Source: CAD feature listing. Evaluate the final solid. Frame: model axes, mm. A direction names the side the tool comes from. Give positions to 0.01 mm unless a question says otherwise; leave off trailing zeros. Write each loop counter-clockwise with the first axis right and the second up, starting at its lowest first coordinate (ties: lowest second). Pieces come first, ordered by that corner, then holes. Notation, with made-up numbers: (40, 20.25) -> (67, 20.25) arc R31 cw to (67, 51.25) -> close; hole circle Ø5 at (3, 29.5). An arc over 180 degrees is marked (long way). Write item = value, one per line.
from build123d import *

# Parameters (mm, degrees)
SKETCH_R        = 1.95
SKETCH_W        = 6.8
SKETCH_H        = 46.08113
PAD_DEPTH       = 3
SKETCH001_W     = 22
SKETCH001_H     = 72
PAD001_DEPTH    = 6.5
SKETCH002_W     = 8
SKETCH002_H     = 40
PAD002_DEPTH    = 7.5
SKETCH003_R     = 6.1
POCKET_DEPTH    = 3.5
SKETCH004_R     = 3
POCKET001_DEPTH = 6.5
CHAMFER_SIZE    = 3
CHAMFER001_SIZE = 0.5


with BuildPart() as part:
    # Sketch → Pad (new body)
    with BuildSketch(Plane.XY):
        Polygon((54.045437, 24.98), (101.633751, 24.98), (101.633751, -24.98), (54.045437, -24.98), (43.025437, -36), (0, -36), (0, 36), (43.025437, 36), align=None)
        with Locations((42.6, 21.78)):
            Circle(SKETCH_R, mode=Mode.SUBTRACT)
        with Locations((42.6, -21.78)):
            Circle(SKETCH_R, mode=Mode.SUBTRACT)
        with Locations((96.7, 21.78)):
            Circle(SKETCH_R, mode=Mode.SUBTRACT)
        with Locations((96.7, -21.78)):
            Circle(SKETCH_R, mode=Mode.SUBTRACT)
        with Locations((35.4, 0)):
            Rectangle(SKETCH_W, SKETCH_H, mode=Mode.SUBTRACT)
    extrude(amount=PAD_DEPTH)

    # Sketch001 → Pad001 (join)
    with BuildSketch(Plane.XY):
        with Locations((11, 0)):
            Rectangle(SKETCH001_W, SKETCH001_H)
    extrude(amount=PAD001_DEPTH)

    # Sketch002 → Pad002 (join)
    with BuildSketch(Plane.XY):
        with Locations((14, 0)):
            Rectangle(SKETCH002_W, SKETCH002_H)
    extrude(amount=PAD002_DEPTH)

    # Sketch003 → Pocket (cut)
    with BuildSketch(Plane.XY):
        with Locations((14, 25)):
            Circle(SKETCH003_R)
        with Locations((14, -25)):
            Circle(SKETCH003_R)
    extrude(amount=POCKET_DEPTH, mode=Mode.SUBTRACT)

    # Sketch004 → Pocket001 (cut)
    with BuildSketch(Plane.XY):
        with Locations((14, 25)):
            Circle(SKETCH004_R)
        with Locations((14, -25)):
            Circle(SKETCH004_R)
    extrude(amount=POCKET001_DEPTH, mode=Mode.SUBTRACT)

    # Chamfer
    chamfer_edges = [part.edges().sort_by_distance(p)[0] for p in [
        (101.633751, -24.98, 1.5),
        (101.633751, 24.98, 1.5),
        (22, 36, 4.75),
        (0, 36, 1.5),
        (0, 36, 4.75),
        (0, -36, 4.75),
        (0, -36, 1.5),
        (22, -36, 4.75),
    ]]
    chamfer(chamfer_edges, length=CHAMFER_SIZE)

    # Chamfer001
    chamfer001_edges = [part.edges().sort_by_distance(p)[0] for p in [
        (48.535437, 30.49, 3),
        (76.339594, 24.98, 3),
        (100.133751, 23.48, 3),
        (101.633751, 0, 3),
        (100.133751, -23.48, 3),
        (76.339594, -24.98, 3),
        (76.339594, -24.98, 0),
        (48.535437, -30.49, 3),
        (48.535437, -30.49, 0),
        (32.512719, -36, 0),
        (32.512719, -36, 3),
        (1.5, -34.5, 0),
        (0, 0, 0),
        (1.5, 34.5, 6.5),
        (32.512719, 36, 3),
        (11, 36, 6.5),
        (1.5, 34.5, 0),
        (12.5, 36, 0),
        (100.133751, -23.48, 0),
        (76.339594, 24.98, 0),
        (22, 0, 6.5),
        (44.55, 21.78, 1.5),
        (20.5, 34.5, 6.5),
        (20.5, -36, 3),
        (0, 0, 6.5),
        (12.5, -36, 0),
        (20.5, 36, 3),
        (32.512719, 36, 0),
        (48.535437, 30.49, 0),
        (100.133751, 23.48, 0),
        (101.633751, 0, 0),
        (20.5, -34.5, 6.5),
        (11, -36, 6.5),
        (1.5, -34.5, 6.5),
    ]]
    chamfer(chamfer001_edges, length=CHAMFER001_SIZE)


solid = part.part
(1) Section query A-A (z = 5). Return loops of the section in (x, y).
Values follow:
outline = (0, -33) -> (3, -36) -> (19, -36) -> (22, -33) -> (22, 33) -> (19, 36) -> (3, 36) -> (0, 33) -> close; hole circle Ø6 at (14, -25); hole circle Ø6 at (14, 25)
(2) Section query C-C (y = -27). Return loops of the section in (x, z), plus the area to 3 significant figures.
Values follow:
outline = (0, 0.5) -> (0.5, 0) -> (8.24, 0) -> (8.24, 3.5) -> (11.76, 3.5) -> (11.76, 6.5) -> (0.5, 6.5) -> (0, 6) -> close; (16.24, 3.5) -> (19.76, 3.5) -> (19.76, 0) -> (51.32, 0) -> (52.03, 0.5) -> (52.03, 2.5) -> (51.32, 3) -> (22, 3) -> (22, 6) -> (21.5, 6.5) -> (16.24, 6.5) -> close
area = 179 mm2
(3) First-contact query: pin 1 (12 mm diameter, centred on x = 43.5, y = -4.5, fed in from +Z); pin 2 (7.5 mm diameter, centred on x = 14, y = 25, fed in from +Z); pin 3 (3 mm diameter, centred on y = -2.5, z = 6.5, fed in from -X); pin 4 (5.5 mm diameter, centred on x = 14, y = -25, fed in from +Z). Flat tips, straight axial feed; report the tip coordinate or a pass-through.
Values follow:
pin_1 = 3
pin_2 = 6.5
pin_3 = 0
pin_4 = through
(4) Pull-direction query (Y, two-part tool) for faces 4 (the face through (100.155, 23.459, 1.486)), 5 (the face through (97.6, -23.51, 1.48)), 6 (the face through (50, 0, 0)); classes: pulls with the +Y half, pulls with the -Y half, needs draft (parallel to the pull), parting line crosses it, or undercut.
Values follow:
face_4 = pulls with the +Y half
face_5 = undercut
face_6 = needs draft
(5) Section query D-D (x = 37.5). Return loops of the section in (y, z), plus the area to 3 significant figures.
Values follow:
outline = (-36, 0.5) -> (-35.5, 0) -> (-23.04, 0) -> (-23.04, 3) -> (-35.5, 3) -> (-36, 2.5) -> close; (23.04, 0) -> (35.5, 0) -> (36, 0.5) -> (36, 2.5) -> (35.5, 3) -> (23.04, 3) -> close
area = 77.3 mm2
(6) Material intervals for line 1 (Y direction, x = 96.7, z = 1.4); line 2 (Y direction, x = 42.6, z = 1.2); line 3 (X direction, y = 20.5, z = 2.75), sorted ascending.
Values follow:
line_1 = -24.98 to -23.73, -19.83 to 19.83, 23.73 to 24.98
line_2 = -36 to -23.73, -19.83 to 19.83, 23.73 to 36
line_3 = 0 to 9.88, 18.12 to 32, 38.8 to 41.13, 44.07 to 95.23, 98.17 to 101.38
(7) Access query for faces 1 (the face through (22, 0, 4)), 2 (the face through (1, 34, 3)), 3 (the face through (21, -34, 5)). Directions: +Z, -Z, +X, -X, +Y, -Y. A direction counts if a zero-diameter tool reaches every point of the face in a straight line with its end or side. Return the directions, or none.
Values follow:
face_1 = +Z, +X, +Y, -Y
face_2 = +Z, -Z, -X, +Y
face_3 = +Z, +X, -Y
(8) Section query B-B (x = 96.7). Return loops of the section in (y, z), plus the area to 3 significant figures.
Values follow:
outline = (-24.98, 0.5) -> (-24.48, 0) -> (-23.73, 0) -> (-23.73, 3) -> (-24.48, 3) -> (-24.98, 2.5) -> close; (-19.83, 0) -> (19.83, 0) -> (19.83, 3) -> (-19.83, 3) -> close; (23.73, 0) -> (24.48, 0) -> (24.98, 0.5) -> (24.98, 2.5) -> (24.48, 3) -> (23.73, 3) -> close
area = 126 mm2
